The model under review builds one solid part; all positions refer to its coordinate system, in mm. Face numbers are marked on the shaded views. A direction names the side the tool comes from. Round coordinates to 2 decimals unless told otherwise and drop trailing zeros. Order: outer loops, then holes, each group sorted by start corner. A loop starts at its lowest first (then second) coordinate and runs counter-clockwise, first axis right, second up.
from build123d import *

# Parameters (mm, degrees)
EXTRUDE1_DEPTH          = 25.4
F_3_8_CLEARANCE_HOLE1_D = 10.31748
CUT_EXTRUDE1_REACH      = 58.454
SKETCH5_R               = 5.55625


with BuildPart() as part:
    # Sketch1 → Extrude1 (new body)
    with BuildSketch(Plane.XY):
        with BuildLine():
            Line((0, 0), (0, 38.1))
            Line((0, 38.1), (1.905, 38.1))
            ThreePointArc((1.905, 38.1), (4.15006403, 37.17006403), (5.08, 34.925))
            Line((5.08, 34.925), (5.08, 9.8425))
            ThreePointArc((5.08, 9.8425), (6.474903955, 6.474903955), (9.8425, 5.08))
            Line((9.8425, 5.08), (34.925, 5.08))
            ThreePointArc((34.925, 5.08), (37.17006403, 4.15006403), (38.1, 1.905))
            Line((38.1, 1.905), (38.1, 0))
            Line((38.1, 0), (0, 0))
        make_face()
    extrude(amount=EXTRUDE1_DEPTH)

    # 3/8 Clearance Hole1 (through all)
    with Locations(Plane(origin=(0, 5.08, 0), x_dir=(-1, 0, 0), z_dir=(0, 1, 0))):
        with Locations((-19.05, 12.7)):
            Hole(F_3_8_CLEARANCE_HOLE1_D / 2)

    # Sketch5 → Cut-Extrude1 (cut, up to next)
    with BuildSketch(Plane(origin=(5.08, 0, 0), x_dir=(0, 0, -1), z_dir=(1, 0, 0)), mode=Mode.PRIVATE) as cut_extrude1_sk1:
        with Locations(Location((-12.7, 25.4, 0), (0, 0, 90))):
            Circle(SKETCH5_R)
    cut_extrude1_tool1 = extrude(cut_extrude1_sk1.sketch, amount=-CUT_EXTRUDE1_REACH, mode=Mode.PRIVATE) & part.part
    add(cut_extrude1_tool1.solids().sort_by_distance((5.08, 25.4, 12.7))[0], mode=Mode.SUBTRACT)


solid = part.part
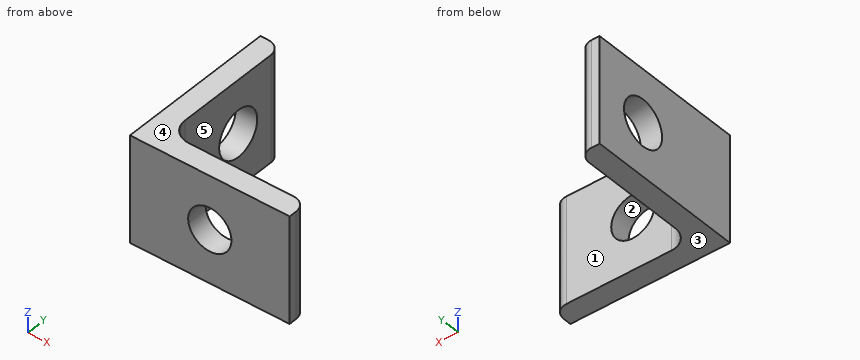
(1) To check wall thickness, follow L1, parallel to Z at x = 19.05, y = 2.6; L2, parallel to Z at x = 2.65, y = 25.4; L3, parallel to Y at x = 27, z = 23.5. State the ranges of each line that lie inside material, in increasing order.
(2) We need section A-A (z = 12.7). Count the separate pieces of the cut face and the enclosed holes in it, and give its area (3 significant figures).
(3) Clearance check with flat-ended pins moving along their axes: P1, Ø1.5, axis at y = 14.5, z = 21, coming from the +X side; P2, Ø10, axis at x = 18.5, z = 2.5, coming from the +Y side. State where each tip first meets the part, or that it passes through.
(4) We need section B-B (x = 19.05). Give the boundary of the cut face in (y, z), and give its area (3 significant figures).
(5) We need section C-C (y = 25.4). Give the boundary of the cut face in (x, z), and give its area (3 significant figures).
(6) Tool access review of the marked faces 4 and 5: name each direction out of +Z, -Z, +X, -X, +Y, -Y from which nothing blocks a thin tool from reaching the whole face with its end or side.
(7) The part is to be moulded in two halves that separate along Z. For the marked faces 1, 2 and 3, say which applies: pulls with the +Z half, pulls with the -Z half, needs draft (parallel to the pull), parting line crosses it, or undercut.
Verdict:
1. L1: z = 0 to 7.54, 17.86 to 25.4
1. L2: z = 0 to 7.14, 18.26 to 25.4
1. L3: y = 0 to 5.08
2. separate pieces: 3
2. enclosed holes: 0
2. area: 253 mm2
3. P1: stops at x = 5.08
3. P2: stops at y = 5.08
4. outline: (0, 0) - (5.08, 0) - (5.08, 7.54) - (0, 7.54) - close; (0, 17.86) - (5.08, 17.86) - (5.08, 25.4) - (0, 25.4) - close
4. area: 76.6 mm2
5. outline: (0, 0) - (5.08, 0) - (5.08, 7.14) - (0, 7.14) - close; (0, 18.26) - (5.08, 18.26) - (5.08, 25.4) - (0, 25.4) - close
5. area: 72.6 mm2
6. face 4: +Z, +X, -X, +Y, -Y
6. face 5: +Z, -Z, +X, +Y
7. face 1: needs draft
7. face 2: undercut
7. face 3: pulls with the -Z half
